```python
from build123d import *

# Parameters (mm, degrees)
BOSS_EXTRUDE1_DEPTH = 50.8
CUT_EXTRUDE1_DEPTH  = 40
CUT_EXTRUDE2_DEPTH  = 50.8
SKETCH4_R           = 1.65
CUT_EXTRUDE3_DEPTH  = 25.4


with BuildPart() as part:
    # Sketch1 → Boss-Extrude1 (new body)
    with BuildSketch(Plane(origin=(0, 0, 0), x_dir=(1, 0, 0), z_dir=(0, 1, 0))):
        Polygon((0, 0), (-4.47870531, 25.4), (10, 25.4), (10, 0), align=None)
    extrude(amount=BOSS_EXTRUDE1_DEPTH)

    # Sketch2 → Cut-Extrude1 (cut)
    with BuildSketch(Plane.XZ):
        Polygon((10, -25.4), (-4.47870531, -25.4), (-1.763269807, -10), (10, -10), align=None)
    extrude(amount=-CUT_EXTRUDE1_DEPTH, mode=Mode.SUBTRACT)

    # Sketch3 → Cut-Extrude2 (cut)
    with BuildSketch(Plane(origin=(0, 0, 0), x_dir=(-1, 0, 0), z_dir=(0, -1, 0))):
        Polygon((-10, 2.5), (0.440817452, 2.5), (0, 0), (-10, 0), align=None)
    extrude(amount=-CUT_EXTRUDE2_DEPTH, mode=Mode.SUBTRACT)

    # Sketch4 → Cut-Extrude3 (cut)
    with BuildSketch(Plane(origin=(0, 40, 0), x_dir=(-1, 0, 0), z_dir=(0, -1, 0))):
        with Locations(Location((-3.18210765, 16.56485457, 0), (0, 0, 90))):
            Circle(SKETCH4_R)
        with Locations(Location((-2.278142793, 12.66833721, 0), (0, 0, 90))):
            Circle(SKETCH4_R)
    extrude(amount=-CUT_EXTRUDE3_DEPTH, mode=Mode.SUBTRACT)


solid = part.part
```
The model under review builds one solid part; all positions refer to its coordinate system, in mm. A direction names the side the tool comes from. Give positions to 0.01 mm unless a question says otherwise; leave off trailing zeros. Order: outer loops, then holes, each group sorted by start corner. A loop starts at its lowest first (then second) coordinate and runs counter-clockwise, first axis right, second up. Notation, with made-up numbers: (-31, 18.5) - (-20, 18.5) arc R25 cw to (-20, 55.5) - close; hole circle Ø10 at (14.5, 24.25). An arc over 180 degrees is marked (long way). Use CSV: the item, a comma, the result in double quotes. Start each with the question number.
Q1. The part is to be moulded in two halves that separate along X. For faces 1 (the flat face through (5, 25, -2.5)), 2 (the cylindrical face through (2.774, 45.324, -14.242)), 3 (the cylindrical face through (1.72, 45.32, -17.33)), 4 (the flat face through (-1.534, 30.689, -8.701)), say which applies: +X half, -X half, draft (parallel to the pull), parting line (faces both ways), or undercut.
Q2. We need section B-B, the plane x = 8.75. Write out the cut boundary in (y, z), and give its area (3 significant figures).
Q3. Clearance check with flat-ended pins moving along their axes: pin 1 Ø4 at (x, z) = (6.5, -16) entering from -Y; pin 2 Ø3 at (x, y) = (2.5, 15.5) entering from -Z. State where each tip first meets the part, or that it passes through.
Q4. Tool access review of faces 5 (the flat face through (10, 31, -9)), 6 (the flat face through (4, 20, -10)): name each direction out of +Z, -Z, +X, -X, +Y, -Y from which nothing blocks a thin tool from reaching the whole face with its end or side.
Q5. We need section A-A, the plane z = -12. Write out the cut boundary in (x, y), and give its area (3 significant figures).
Q6. We need section C-C, the plane y = 30. Write out the cut boundary in (x, z), and give its area (3 significant figures).
Q7. To check wall thickness, follow line 1 along Z through (x, y) = (3.25, 27); line 2 along Y through (x, z) = (-2, -14.75); line 3 along X through (y, z) = (42.5, -23.5). State the ranges of each line that lie inside material, in increasing order. Write a range as [from, to].
Q8. We need section D-D, the plane z = -17.5. Write out the cut boundary in (x, y).
Outcome:
1,face 1,"draft"
1,face 2,"undercut"
1,face 3,"undercut"
1,face 4,"-X half"
2,outline,"(0, -10) - (40, -10) - (40, -25.4) - (50.8, -25.4) - (50.8, -2.5) - (0, -2.5) - close"
2,area,"547 mm^2"
3,pin 1,"stops at y = 40"
3,pin 2,"stops at z = -10"
4,face 5,"+Z, -Z, +X, +Y, -Y"
4,face 6,"-Z, +X, -X, -Y"
5,outline,"(-2.12, 40) - (0.77, 40) - (0.77, 50.8) - (-2.12, 50.8) - close; (3.79, 40) - (10, 40) - (10, 50.8) - (3.79, 50.8) - close"
5,area,"98.3 mm^2"
6,outline,"(-1.76, -10) - (10, -10) - (10, -2.5) - (-0.44, -2.5) - close"
6,area,"83.3 mm^2"
7,line 1,"z = [-10, -2.5]"
7,line 2,"y = [40, 50.8]"
7,line 3,"x = [-4.14, 10]"
8,outline,"(-3.09, 40) - (1.82, 40) - (1.82, 50.8) - (-3.09, 50.8) - close; (4.54, 40) - (10, 40) - (10, 50.8) - (4.54, 50.8) - close"
